For this review, use the dimensioned drawing (mm, ordinates from the lowest corner) and the shaded views. A direction names the side the tool comes from. Give positions to 0.01 mm unless a question says otherwise; leave off trailing zeros. Order: outer loops, then holes, each group sorted by start corner. A loop starts at its lowest first (then second) coordinate and runs counter-clockwise, first axis right, second up.
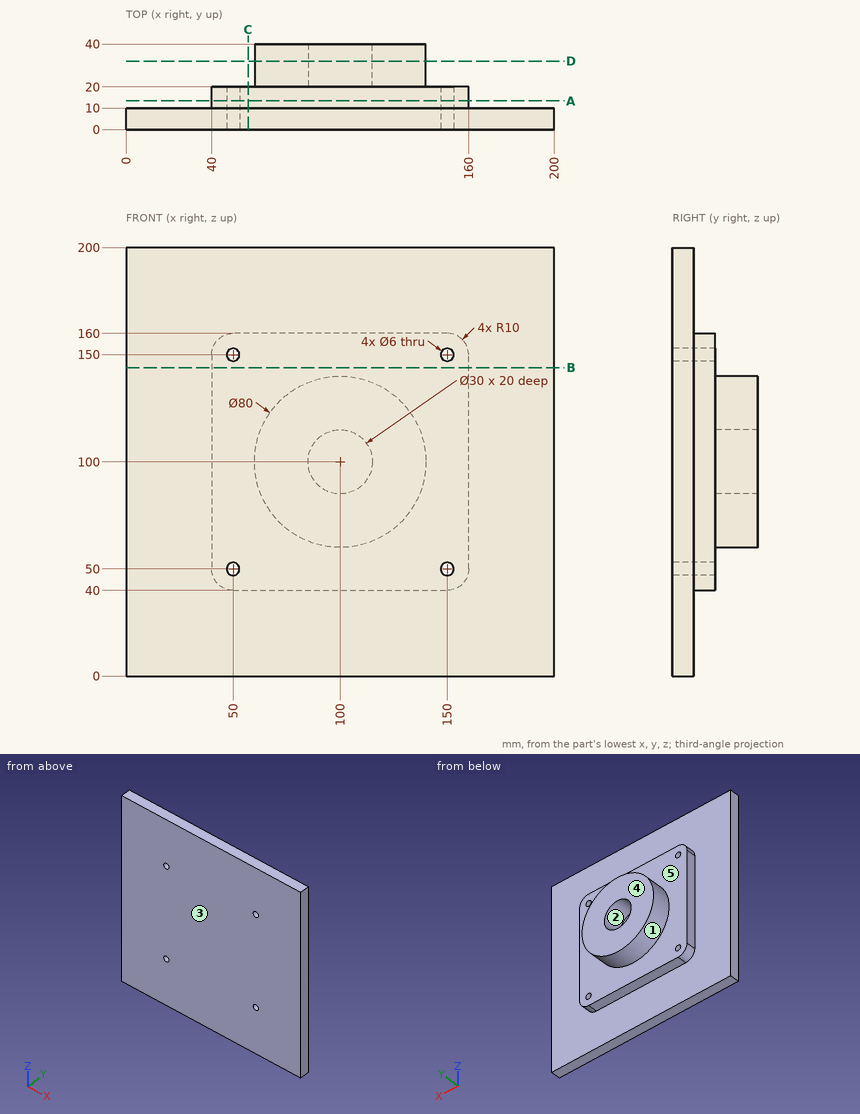
1. Take a section at D-D (y = 32). State the section outline as (x, z) points, then the cut area to 3 significant figures.
Recorded:
outline: circle Ø80 at (100, 100); hole circle Ø30 at (100, 100)
area: 4,320 mm2
2. Machinability: for the marked faces 4 and 5, which of the approach directions +Z, -Z, +X, -X, +Y, -Y give a long, thin tool a straight path to every point of the face, cutting with its end or side? Answer none if there is none.
Recorded:
face 4: +Z, -Z, +X, -X, +Y
face 5: +Y
3. For pin 1 (8 mm diameter, centred on x = 113, y = 13.5, fed in from -Z); pin 2 (7 mm diameter, centred on x = 50, z = 50, fed in from +Y); pin 3 (3 mm diameter, centred on y = 17.5, z = 105, fed in from +X); pin 4 (1 mm diameter, centred on x = 172.5, z = 47.5, fed in from +Y), all flat-tipped, find the tip position at first contact; note any pin that passes through.
Recorded:
pin 1: stops at z = 0
pin 2: stops at y = 20
pin 3: stops at x = 160
pin 4: stops at y = 10
4. Take a section at C-C (x = 57). State the section outline as (y, z) points, then the cut area to 3 significant figures.
Recorded:
outline: (0, 0) - (10, 0) - (10, 40) - (20, 40) - (20, 160) - (10, 160) - (10, 200) - (0, 200) - close
area: 3,200 mm2
5. Take a section at B-B (z = 144). State the section outline as (x, y) points, then the cut area to 3 significant figures.
Recorded:
outline: (0, 0) - (200, 0) - (200, 10) - (160, 10) - (160, 20) - (40, 20) - (40, 10) - (0, 10) - close
area: 3,200 mm2
6. Draft analysis for pull direction Z (two halves, no side actions). For the marked faces 1, 2 and 3, state which applies: pulls with the +Z half, pulls with the -Z half, needs draft (parallel to the pull), parting line crosses it, or undercut.
Recorded:
face 1: parting line crosses it
face 2: undercut
face 3: needs draft
7. For line 1 along Z through (x, y) = (150, 11); line 2 along X through (y, z) = (7.5, 150), list the stretches that pass through material, from the lowest coordinate up.
Recorded:
line 1: z = 40 to 47, 53 to 147, 153 to 160
line 2: x = 0 to 47, 53 to 147, 153 to 200
8. Take a section at A-A (y = 13.5). State the section outline as (x, z) points, then the cut area to 3 significant figures.
Recorded:
outline: (40, 50) arc R10 ccw to (50, 40) - (150, 40) arc R10 ccw to (160, 50) - (160, 150) arc R10 ccw to (150, 160) - (50, 160) arc R10 ccw to (40, 150) - close; hole circle Ø6 at (50, 50); hole circle Ø6 at (50, 150); hole circle Ø6 at (150, 50); hole circle Ø6 at (150, 150)
area: 14,200 mm2
